CAD build for the part. Positions are in the model's coordinates, mm. A direction names the side the tool comes from. Round coordinates to 2 decimals unless told otherwise and drop trailing zeros. Order: outer loops, then holes, each group sorted by start corner. A loop starts at its lowest first (then second) coordinate and runs counter-clockwise, first axis right, second up. Notation, with made-up numbers: M 29,1.25 L 42,1.25 A27 cw 42,36.25 Z; hole C -13.75,-13 d8. An arc over 180 degrees is marked long. Answer as a JSON object with one key per item and string values.
```python
from build123d import *

# Parameters (mm, degrees)
BOSS_EXTRUDE3_DEPTH = 15.24
SKETCH6_R           = 3.175
CUT_EXTRUDE2_DEPTH  = 16.24
CUT_EXTRUDE6_REACH  = 17.24
SKETCH53_R          = 2.413
FILLET1_R           = 3.81
SKETCH57_R          = 3.96875
CUT_EXTRUDE8_DEPTH  = 11.43
SKETCH55_R          = 3.96875
CUT_EXTRUDE9_DEPTH  = 11.43
CIRPATTERN2_COUNT   = 4
SKETCH59_R          = 2.605475785
CUT_EXTRUDE11_DEPTH = 6.35
SKETCH60_R          = 2.660599197
CUT_EXTRUDE12_DEPTH = 6.35
SKETCH62_R          = 2.54
CUT_EXTRUDE14_DEPTH = 3.81


with BuildPart() as part:
    # Sketch5 → Boss-Extrude3 (new body)
    with BuildSketch(Plane(origin=(0, 0, 0), x_dir=(1, 0, 0), z_dir=(0, 1, 0))):
        with BuildLine():
            Line((-11.833206742, -44.162128778), (-88.108068982, -120.436991017))
            ThreePointArc((-88.108068982, -120.436991017), (-105.518009423, -105.518009423), (-120.436991017, -88.108068982))
            Line((-120.436991017, -88.108068982), (-44.162128778, -11.833206742))
            ThreePointArc((-44.162128778, -11.833206742), (-45.72, 0), (-44.162128778, 11.833206742))
            Line((-44.162128778, 11.833206742), (-120.436991017, 88.108068982))
            ThreePointArc((-120.436991017, 88.108068982), (-105.518009423, 105.518009423), (-88.108068982, 120.436991017))
            Line((-88.108068982, 120.436991017), (-11.833206742, 44.162128778))
            ThreePointArc((-11.833206742, 44.162128778), (0, 45.72), (11.833206742, 44.162128778))
            Line((11.833206742, 44.162128778), (88.108068982, 120.436991017))
            ThreePointArc((88.108068982, 120.436991017), (105.518009423, 105.518009423), (120.436991017, 88.108068982))
            Line((120.436991017, 88.108068982), (44.162128778, 11.833206742))
            ThreePointArc((44.162128778, 11.833206742), (45.72, 0), (44.162128778, -11.833206742))
            Line((44.162128778, -11.833206742), (120.436991017, -88.108068982))
            ThreePointArc((120.436991017, -88.108068982), (105.518009423, -105.518009423), (88.108068982, -120.436991017))
            Line((88.108068982, -120.436991017), (11.833206742, -44.162128778))
            ThreePointArc((11.833206742, -44.162128778), (0, -45.72), (-11.833206742, -44.162128778))
        make_face()
    extrude(amount=BOSS_EXTRUDE3_DEPTH)

    # Sketch6 → Cut-Extrude2 (cut, through all)
    with BuildSketch(Plane(origin=(0, 15.24, 0), x_dir=(1, 0, 0), z_dir=(0, 1, 0))):
        with Locations((-74.536125805, -94.292689271)):
            Circle(SKETCH6_R)
        with Locations((-94.292689271, -74.536125805)):
            Circle(SKETCH6_R)
        with Locations((94.292689271, -74.536125805)):
            Circle(SKETCH6_R)
        with Locations((74.536125805, -94.292689271)):
            Circle(SKETCH6_R)
        with Locations((94.292689271, 74.536125805)):
            Circle(SKETCH6_R)
        with Locations((74.536125805, 94.292689271)):
            Circle(SKETCH6_R)
        with Locations((-94.292689271, 74.536125805)):
            Circle(SKETCH6_R)
        with Locations((-74.536125805, 94.292689271)):
            Circle(SKETCH6_R)
    extrude(amount=-CUT_EXTRUDE2_DEPTH, mode=Mode.SUBTRACT)

    # Sketch53 → Cut-Extrude6 (cut, up to next)
    with BuildSketch(Plane(origin=(0, 15.24, 0), x_dir=(1, 0, 0), z_dir=(0, 1, 0)), mode=Mode.PRIVATE) as cut_extrude6_sk1:
        with Locations((-88.455522793, -101.027881362)):
            Circle(SKETCH53_R)
    cut_extrude6_tool1 = extrude(cut_extrude6_sk1.sketch, amount=-CUT_EXTRUDE6_REACH, mode=Mode.PRIVATE) & part.part
    add(cut_extrude6_tool1.solids().sort_by_distance((-88.455523, 15.24, 101.027881))[0], mode=Mode.SUBTRACT)
    # Sketch53 → Cut-Extrude6 (cut, up to next)
    with BuildSketch(Plane(origin=(0, 15.24, 0), x_dir=(1, 0, 0), z_dir=(0, 1, 0)), mode=Mode.PRIVATE) as cut_extrude6_sk2:
        with Locations((-52.534498308, -65.106856878)):
            Circle(SKETCH53_R)
    cut_extrude6_tool2 = extrude(cut_extrude6_sk2.sketch, amount=-CUT_EXTRUDE6_REACH, mode=Mode.PRIVATE) & part.part
    add(cut_extrude6_tool2.solids().sort_by_distance((-52.534498, 15.24, 65.106857))[0], mode=Mode.SUBTRACT)
    # Sketch53 → Cut-Extrude6 (cut, up to next)
    with BuildSketch(Plane(origin=(0, 15.24, 0), x_dir=(1, 0, 0), z_dir=(0, 1, 0)), mode=Mode.PRIVATE) as cut_extrude6_sk3:
        with Locations((-101.925906974, -87.55749718)):
            Circle(SKETCH53_R)
    cut_extrude6_tool3 = extrude(cut_extrude6_sk3.sketch, amount=-CUT_EXTRUDE6_REACH, mode=Mode.PRIVATE) & part.part
    add(cut_extrude6_tool3.solids().sort_by_distance((-101.925907, 15.24, 87.557497))[0], mode=Mode.SUBTRACT)
    # Sketch53 → Cut-Extrude6 (cut, up to next)
    with BuildSketch(Plane(origin=(0, 15.24, 0), x_dir=(1, 0, 0), z_dir=(0, 1, 0)), mode=Mode.PRIVATE) as cut_extrude6_sk4:
        with Locations((-66.00488249, -51.636472696)):
            Circle(SKETCH53_R)
    cut_extrude6_tool4 = extrude(cut_extrude6_sk4.sketch, amount=-CUT_EXTRUDE6_REACH, mode=Mode.PRIVATE) & part.part
    add(cut_extrude6_tool4.solids().sort_by_distance((-66.004882, 15.24, 51.636473))[0], mode=Mode.SUBTRACT)

    # Fillet1
    fillet1_edges = [part.edges().sort_by_distance(p)[0] for p in [
        (-44.162128778, 7.62, 11.833206742),
        (-44.162128778, 7.62, -11.833206742),
        (-11.833206742, 7.62, -44.162128778),
        (11.833206742, 7.62, -44.162128778),
        (44.162128778, 7.62, -11.833206742),
        (44.162128778, 7.62, 11.833206742),
        (11.833206742, 7.62, 44.162128778),
        (-11.833206742, 7.62, 44.162128778),
    ]]
    fillet(fillet1_edges, radius=FILLET1_R)

    # Sketch57 → Cut-Extrude8 (cut)
    with BuildSketch(Plane(origin=(-114.312982024, 0, 95.919981055), x_dir=(0.64278761, 0, 0.766044443), z_dir=(-0.766044443, 0, 0.64278761))):
        with Locations((0, 7.62)):
            Circle(SKETCH57_R)
    cut_extrude8 = extrude(amount=-CUT_EXTRUDE8_DEPTH, mode=Mode.SUBTRACT)

    # Sketch55 → Cut-Extrude9 (cut)
    with BuildSketch(Plane(origin=(-95.919981055, 0, 114.312982024), x_dir=(0.766044443, 0, 0.64278761), z_dir=(-0.64278761, 0, 0.766044443))):
        with Locations((0, 7.62)):
            Circle(SKETCH55_R)
    cut_extrude9 = extrude(amount=-CUT_EXTRUDE9_DEPTH, mode=Mode.SUBTRACT)

    # CirPattern2: Cut-Extrude8, Cut-Extrude9 ×4 about axis
    cirpattern2_axis = Axis((0, 0, 0), (0, 1, 0))
    for i in range(1, CIRPATTERN2_COUNT):
        add(cut_extrude8.rotate(cirpattern2_axis, i * 360 / CIRPATTERN2_COUNT), mode=Mode.SUBTRACT)
        add(cut_extrude9.rotate(cirpattern2_axis, i * 360 / CIRPATTERN2_COUNT), mode=Mode.SUBTRACT)

    # Sketch59 → Cut-Extrude11 (cut)
    with BuildSketch(Plane(origin=(-16.164461018, 0, -16.164461018), x_dir=(-0.707106781, 0, 0.707106781), z_dir=(-0.707106781, 0, -0.707106781))):
        with Locations((-75.363184789, 6.985)):
            Circle(SKETCH59_R)
    extrude(amount=-CUT_EXTRUDE11_DEPTH, mode=Mode.SUBTRACT)

    # Sketch60 → Cut-Extrude12 (cut)
    with BuildSketch(Plane(origin=(16.164461018, 0, 16.164461018), x_dir=(0.707106781, 0, -0.707106781), z_dir=(0.707106781, 0, 0.707106781))):
        with Locations((75.363184789, 6.985)):
            Circle(SKETCH60_R)
    extrude(amount=-CUT_EXTRUDE12_DEPTH, mode=Mode.SUBTRACT)

    # Sketch62 → Cut-Extrude14 (cut)
    with BuildSketch(Plane.XZ):
        with Locations((93.894945093, -94.405023641)):
            Circle(SKETCH62_R)
    extrude(amount=-CUT_EXTRUDE14_DEPTH, mode=Mode.SUBTRACT)


solid = part.part
```
Item 1: Two-plate mould, pull along Y, no slides. Class faces 1 (the cylindrical face through (65.36, 7.1, -37.46)), 2 (the cylindrical face through (-96.633, 7.727, -76.682)): released by +Y, released by -Y, zero draft, split by the parting line, or undercut.
Worked answers:
{"face 1": "undercut", "face 2": "zero draft"}
Item 2: Drop flat-ended pins along their axis: pin 1 Ø2.5 at (x, z) = (95, -94.5) entering from -Y; pin 2 Ø4 at (x, z) = (-101.93, 87.56) entering from -Y; pin 3 Ø1 at (x, y) = (94, 2) entering from +Z; pin 4 Ø8 at (x, y) = (59.5, 13) entering from +Z. Give the stop position or say it passes through.
Worked answers:
{"pin 1": "stops at y = 3.81", "pin 2": "passes through", "pin 3": "stops at z = 116.3", "pin 4": "stops at z = 95.83"}
Item 3: Saw through at B-B on x = -37. List the corners of the cut face in (y, z).
Worked answers:
{"outline": "M 0,-69.33 L 15.24,-69.33 L 15.24,69.33 L 0,69.33 Z"}
Item 4: 3-axis set-ups, long thin cutter, end or side, ignore diameter. For faces 3 (the flat face through (88.62, 7.68, -105.52)), 4 (the flat face through (-51.25, 7.51, -83.58)), 5 (the flat face through (-50.2, 7.51, 82.53)), 6 (the flat face through (-82.53, 7.51, -50.2)): which of +Z, -Z, +X, -X, +Y, -Y reach the whole face in a straight line?
Worked answers:
{"face 3": "none", "face 4": "-Z, +Y, -Y", "face 5": "+Z, +Y, -Y", "face 6": "-X, +Y, -Y"}
Item 5: Saw through at C-C on z = 16.5. List the corners of the cut face in (x, y).
Worked answers:
{"outline": "M -48.83,0 L 48.83,0 L 48.83,15.24 L -48.83,15.24 Z"}
Item 6: Saw through at A-A on z = 82. List the corners of the cut face in (x, y).
Worked answers:
{"outline": "M -114.33,0 L -49.67,0 L -49.67,15.24 L -114.33,15.24 Z; M 49.67,0 L 114.33,0 L 114.33,15.24 L 49.67,15.24 Z"}
Item 7: Wall check: line 1 along X through (y, z) = (5.5, 50.5); line 2 along Z through (x, y) = (-94.5, 10.25); line 3 along Z through (x, y) = (-68, 12.5). Give the ranges that are in metal, low to high. Write a range as [from, to].
Worked answers:
{"line 1": "x = [-82.83, -68.13], [-63.88, -18.17], [18.17, 82.83]", "line 2": "z = [-108, -77.7], [-71.37, -62.17], [62.17, 71.37], [77.7, 108]", "line 3": "z = [-100.33, -35.67], [35.67, 50.28], [52.99, 100.33]"}
